Study the drawing (mm; zero at the part's minimum x, y, z) and answer. A direction names the side the tool comes from. Coordinates: 2 decimals unless noted, no trailing zeros. Order: outer loops, then holes, each group sorted by start corner. A loop starts at its lowest first (then second) coordinate and runs counter-clockwise, first axis right, second up. Notation, with made-up numbers: (56, 83.25) -> (92, 83.25) arc R24 cw to (92, 107.25) -> close; hole circle Ø6 at (-30.5, 40). An arc over 180 degrees is marked (long way). Write each question's results on one line, items separated by ' | '. Start each with the question number.
(1) Given pin 1 (1.9 mm diameter, centred on x = 95.25, z = 17.11, fed in from -Y); pin 2 (6 mm diameter, centred on x = 29.5, y = 9.5, fed in from +Z); pin 3 (7 mm diameter, centred on x = 98.5, z = 8.5, fed in from +Y), each flat-ended and moving along its own axis, determine where each tip first touches the part or whether it passes through.
(2) The part is cut by section A-A, the plane x = 54. Give the vertices of the cut face in (y, z).
(3) Straight lines are drawn through the part: L1, parallel to Z at x = 95.25, y = 1 (1 decimal); L2, parallel to Z at x = 127, y = 9.5. For each, find the intervals that lie inside material, in ascending order.
(4) A tool of negligible diameter and unlimited length cuts with its end or side. For the marked faces 1 and 2, from which of +Z, -Z, +X, -X, +Y, -Y can it reach the whole face along a straight path? Write none if from no direction.
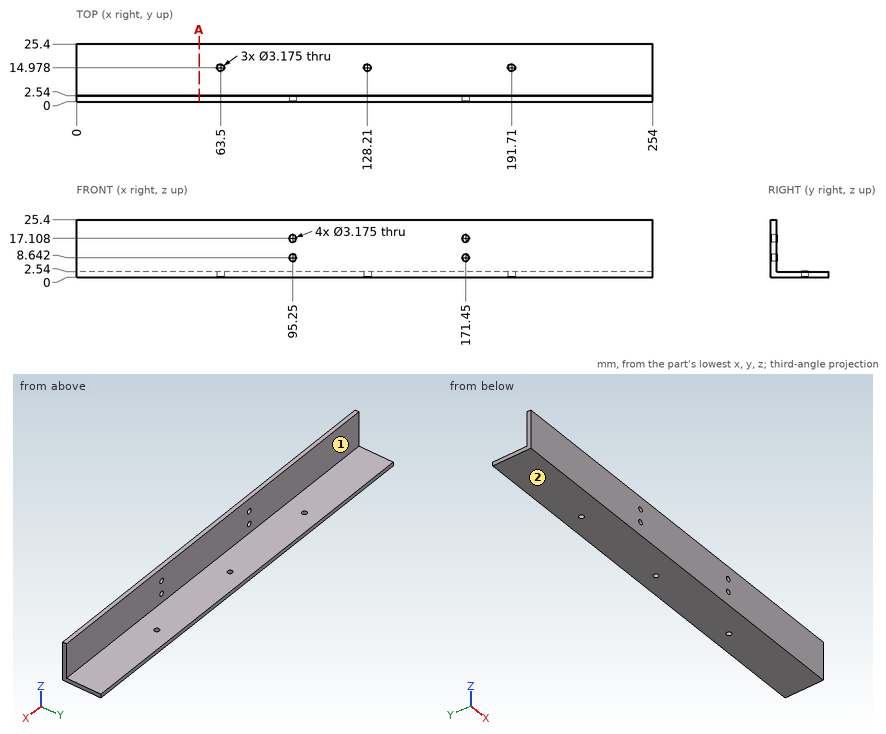
Established:
1) pin 1: passes through | pin 2: stops at z = 2.54 | pin 3: stops at y = 2.54
2) outline: (0, 0) -> (25.4, 0) -> (25.4, 2.54) -> (2.54, 2.54) -> (2.54, 25.4) -> (0, 25.4) -> close
3) L1: z = 0 to 7.1, 10.2 to 15.5, 18.7 to 25.4 | L2: z = 0 to 2.54
4) face 1: +Z, +X, -X, +Y | face 2: -Z, +X, -X, +Y, -Y
